Verification items for the finished model (mm, model axes). A direction names the side the tool comes from. Round coordinates to 2 decimals unless told otherwise and drop trailing zeros. Write each loop counter-clockwise with the first axis right and the second up, starting at its lowest first coordinate (ties: lowest second). Pieces come first, ordered by that corner, then holes.
from build123d import *

# Parameters (mm, degrees)
SKETCH5_R               = 19.05
BOSS_EXTRUDE1_DEPTH     = 11.43
BOSS_EXTRUDE4_REACH     = 13.989
SKETCH12_R              = 19.05
SKETCH12_R_2            = 13.981282801
SKETCH11_R              = 17.145
CUT_EXTRUDE5_DEPTH      = 8.89
SKETCH13_R              = 9.525
CUT_EXTRUDE7_DEPTH      = 6.35
CUT_EXTRUDE7_TAPER      = 40
SKETCH14_W              = 44.104776143
SKETCH14_H              = 21.741572172
CUT_EXTRUDE8_DEPTH      = 1
CUT_EXTRUDE8_DEPTH_BACK = 24.418912122
FILLET6_R               = 5.08


with BuildPart() as part:
    # Sketch1 → Revolve4 (revolve)
    with BuildSketch(Plane(origin=(0, 0, 0), x_dir=(1, 0, 0), z_dir=(0, 1, 0))):
        with BuildLine():
            Line((22.460516589, 20.486669906), (19.920516589, 20.486669906))
            ThreePointArc((19.920516589, 20.486669906), (26.322608025, 11.119844052), (28.575, 0))
            Line((28.575, 0), (31.909428711, 0))
            Line((31.909428711, 0), (31.909428711, 13.981282801))
            Line((31.909428711, 13.981282801), (22.460516589, 20.486669906))
        make_face()
    revolve(axis=Axis((28.575, 0, 0), (1, 0, 0)))

    # Sketch5 → Boss-Extrude1 (add)
    with BuildSketch(Plane(origin=(31.909428711, 0, 0), x_dir=(0, 0, -1), z_dir=(1, 0, 0))):
        Circle(SKETCH5_R)
    extrude(amount=BOSS_EXTRUDE1_DEPTH)

    # Sketch12 → Boss-Extrude4 (add, up to next)
    with BuildSketch(Plane.ZY.offset(-31.909428711), mode=Mode.PRIVATE) as boss_extrude4_sk1:
        Circle(SKETCH12_R)
        Circle(SKETCH12_R_2, mode=Mode.SUBTRACT)
    boss_extrude4_tool1 = extrude(boss_extrude4_sk1.sketch, amount=BOSS_EXTRUDE4_REACH, mode=Mode.PRIVATE) - part.part
    add(boss_extrude4_tool1.solids().sort_by_distance((31.909429, 0, -18.511185))[0])

    # Sketch11 → Cut-Extrude5 (cut)
    with BuildSketch(Plane(origin=(43.339428711, 0, 0), x_dir=(0, 0, -1), z_dir=(1, 0, 0))):
        Circle(SKETCH11_R)
    extrude(amount=-CUT_EXTRUDE5_DEPTH, mode=Mode.SUBTRACT)

    # Sketch13 → Cut-Extrude7 (cut)
    with BuildSketch(Plane(origin=(34.449428711, 0, 0), x_dir=(0, 0, -1), z_dir=(1, 0, 0))):
        Circle(SKETCH13_R)
    extrude(amount=-CUT_EXTRUDE7_DEPTH, taper=CUT_EXTRUDE7_TAPER, mode=Mode.SUBTRACT)

    # Sketch14 → Cut-Extrude8 (cut, two sides)
    with BuildSketch(Plane(origin=(43.339428711, 0, 0), x_dir=(0, 0, -1), z_dir=(1, 0, 0))) as cut_extrude8_sk:
        with Locations((0.388519875, -10.870786086)):
            Rectangle(SKETCH14_W, SKETCH14_H)
    extrude(amount=CUT_EXTRUDE8_DEPTH, mode=Mode.SUBTRACT)
    extrude(cut_extrude8_sk.sketch, amount=-CUT_EXTRUDE8_DEPTH_BACK, mode=Mode.SUBTRACT)

    # Fillet6
    fillet6_edges = [part.edges().sort_by_distance(p)[0] for p in [
        (34.449428711, 9.525, 0),
    ]]
    fillet(fillet6_edges, radius=FILLET6_R)


solid = part.part
Q1. Tool access check on faces 1 (the conical face through (24.417, 19.135, -0.421)), 2 (the flat face through (34.449, 13, 0)). Record the directions out of +Z, -Z, +X, -X, +Y, -Y that give a thin tool (end or side, any length) a straight path to the whole face; none if there is none.
Recorded:
face 1: +X, +Y
face 2: +X, -Y
Q2. Sectioned sample at B-B (x = 36.75). Enter the section's corners in (y, z) (3 decimals), plus the area to 3 significant figures.
Recorded:
outline: (0, -19.05) arc R19.05 ccw to (0, 19.05) - (0, 17.145) arc R17.145 cw to (0, -17.145) - close
area: 108 mm2
Q3. Material ranges on line 1 along Z through (x, y) = (21.5, 16.25); line 2 along Z through (x, y) = (35.5, 3.75); line 3 along X through (y, z) = (18.5, 5.5), recorded low to high.
Recorded:
line 1: z = -12.48 to -9.5, 9.5 to 12.48
line 2: z = -18.68 to -16.73, 16.73 to 18.68
line 3: x = 21.07 to 24.18
Q4. Depth check by flat-ended pin: P1, Ø2, axis at x = 30.5, z = 16, coming from the +Y side; P2, Ø5, axis at x = 38.5, z = 11, coming from the +Y side; P3, Ø12, axis at x = 37.5, z = 5.5, coming from the -Y side; P4, Ø1, axis at y = 6, z = -12.5, coming from the -X side. Enter the tip coordinate at first touch or a pass-through.
Recorded:
P1: stops at y = 11.74
P2: stops at y = 17.05
P3: stops at y = 0
P4: stops at x = 24.7
Q5. Release check for a two-part mould opening along Z. For faces 3 (the cylindrical face through (21.17, 20.48, -0.45)), 4 (the cylindrical face through (38.96, 17.14, -0.38)), 5 (the flat face through (30, 0, -14)) record: released by +Z, released by -Z, zero draft, split by the parting line, or undercut.
Recorded:
face 3: split by the parting line
face 4: undercut
face 5: zero draft
Q6. Sectioned sample at C-C (x = 23.5). Enter the section's corners in (y, z).
Recorded:
outline: (0, -19.77) arc R19.77 ccw to (0, 19.77) - (0, 16.26) arc R16.26 cw to (0, -16.26) - close
Q7. Sectioned sample at A-A (z = 0). Enter the section's corners in (x, y) (3 decimals), plus the area to 3 significant figures.
Recorded:
outline: (19.921, 20.487) arc R28.575 cw to (28.247, 4.32) - (32.635, 8.002) arc R5.08 ccw to (34.449, 11.894) - (34.449, 17.145) - (43.339, 17.145) - (43.339, 19.05) - (24.547, 19.05) - (22.461, 20.487) - close
area: 134 mm2
